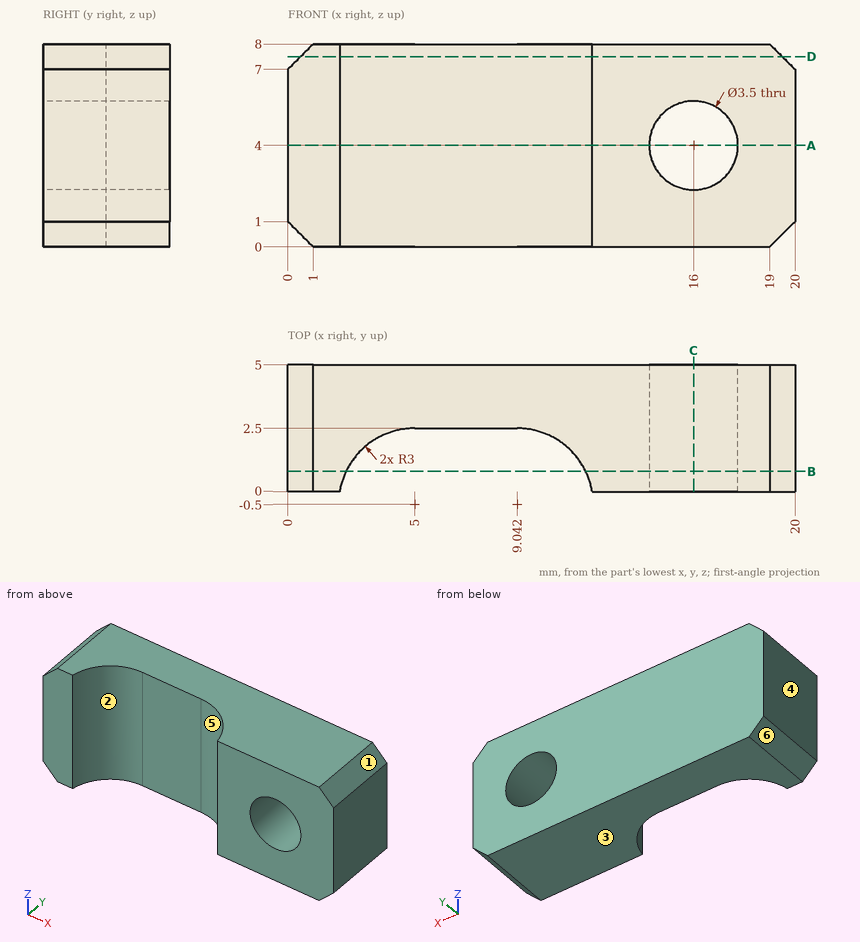
Print and shaded views of the part. All mm, measured from the part's lowest x, y and z. A direction names the side the tool comes from. Round coordinates to 2 decimals unless told otherwise and drop trailing zeros. Write each loop counter-clockwise with the first axis right and the second up, starting at its lowest first coordinate (ties: lowest second). Pieces come first, ordered by that corner, then holes. Notation, with made-up numbers: M -22.75,-2 L -14.75,-2 A16 cw -14.75,7 Z; hole C 82.5,7.25 d8. An arc over 180 degrees is marked long. Use a Markdown table: item, result. Add a question column.
1. Drill centre lines: probe 1 along Z at (x, y) = (16, 1.45); probe 2 along X at (y, z) = (0.5, 5.5); probe 3 along X at (y, z) = (2.1, 3.5). Where is each one in solid material? Low to high.
2. Slice it at C-C on x = 16. Give the cut face in (y, z).
3. Slice it at B-B on y = 0.8. Give the cut face in (x, z), then the cut area to 3 significant figures.
4. Flat gauge pins, fed straight in: P1, Ø4.5, axis at x = 7.5, z = 6, coming from the -Y side; P2, Ø2, axis at x = 7, z = 5.5, coming from the -Y side. Where does each tip first touch, or does it go through?
5. Slice it at A-A on z = 4. Give the cut face in (x, y).
6. 3-axis set-ups, long thin cutter, end or side, ignore diameter. For the marked faces 5 and 6: which of +Z, -Z, +X, -X, +Y, -Y reach the whole face in a straight line?
7. Pull direction X, two halves, no side cores. Call the marked faces 1, 2, 3 and 4: released by +X, released by -X, zero draft, split by the parting line, or undercut.
8. Slice it at D-D on z = 7.5. Give the cut face in (x, y), then the cut area to 3 significant figures.
Reply:
| question | item | result |
|---|---|---|
| 1 | probe 1 | z = 0 to 2.25, 5.75 to 8 |
| 1 | probe 2 | x = 0 to 2.17, 11.87 to 15.1, 16.9 to 20 |
| 1 | probe 3 | x = 0 to 3.5, 10.54 to 14.32, 17.68 to 20 |
| 2 | outline | M 0,0 L 5,0 L 5,2.25 L 0,2.25 Z; M 0,5.75 L 5,5.75 L 5,8 L 0,8 Z |
| 3 | outline | M 0,1 L 1,0 L 2.3,0 L 2.3,8 L 1,8 L 0,7 Z; M 11.75,0 L 19,0 L 20,1 L 20,7 L 19,8 L 11.75,8 Z; hole C 16,4 d3.5 |
| 3 | area | 72.8 mm^2 |
| 4 | P1 | stops at y = 2.42 |
| 4 | P2 | stops at y = 2.5 |
| 5 | outline | M 0,0 L 2.04,0 A3 cw 5,2.5 L 9.04,2.5 A3 cw 12,0 L 14.25,0 L 14.25,5 L 0,5 Z; M 17.75,0 L 20,0 L 20,5 L 17.75,5 Z |
| 6 | face 5 | +Z, -Z, -Y |
| 6 | face 6 | -Z, -X, +Y, -Y |
| 7 | face 1 | released by +X |
| 7 | face 2 | undercut |
| 7 | face 3 | zero draft |
| 7 | face 4 | released by -X |
| 8 | outline | M 0.5,0 L 2.04,0 A3 cw 5,2.5 L 9.04,2.5 A3 cw 12,0 L 19.5,0 L 19.5,5 L 0.5,5 Z |
| 8 | area | 73.7 mm^2 |
